Geometry: final body of the model. Coordinates: model frame, mm. Face numbers are marked on the shaded views. Give positions to 0.01 mm unless a question says otherwise; leave off trailing zeros. Loops run counter-clockwise (first coordinate to the right, second up) from the corner with the lowest first, then second, coordinate; pieces in that order, holes last. Notation, with made-up numbers: M -17,64 L 35,64 A16 cw 35,73 Z; hole C 69.25,84.25 d8. An arc over 180 degrees is marked long. Put each result on its own line as item: value.
```python
from build123d import *

# Parameters (mm, degrees)
SKETCH1_R         = 3.175
CENTER_ROD_DEPTH  = 119.888
CIRCLE_ENDS_DEPTH = 3.175


with BuildPart() as part:
    # Sketch1 → center rod (new body)
    with BuildSketch(Plane(origin=(0, 0, 0), x_dir=(1, 0, 0), z_dir=(0, 1, 0))):
        with Locations(Location((0, 0, 0), (0, 0, 270))):
            Circle(SKETCH1_R)
    extrude(amount=CENTER_ROD_DEPTH)

    # Sketch2 → circle ends (add, symmetric)
    with BuildSketch(Plane.XY):
        with BuildLine():
            Line((-3.175, 119.888), (3.175, 119.888))
            ThreePointArc((3.175, 119.888), (0, 131.737261314), (-3.175, 119.888))
        make_face()
        with BuildLine():
            Line((-3.175, 0), (3.175, 0))
            ThreePointArc((3.175, 0), (0, -11.849261314), (-3.175, 0))
        make_face()
    extrude(amount=CIRCLE_ENDS_DEPTH, both=True)


solid = part.part
```
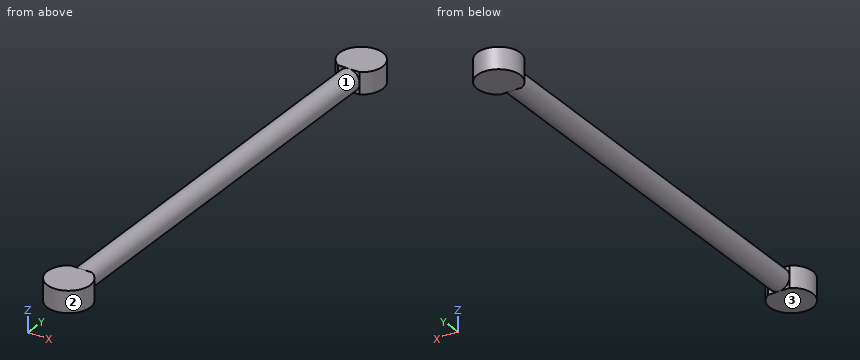
Item 1: Section A-A on x = -5. Output: boundary loops of the cut face in (y, z) (3 decimals), then the cut area to 3 significant figures.
Output values:
outline: M -9.414,-3.175 L -1.585,-3.175 L -1.585,3.175 L -9.414,3.175 Z; M 121.473,-3.175 L 129.302,-3.175 L 129.302,3.175 L 121.473,3.175 Z
area: 99.4 mm²
Item 2: Section B-B on y = 67. Output: boundary loops of the cut face in (x, z) (3 decimals).
Output values:
outline: C 0,0 d6.35
Item 3: Pin query (flat end, axial travel): pin 1 Ø1 at (x, z) = (-1.5, 1) entering from -Y; pin 2 Ø1.6 at (x, z) = (-1.5, -2.5) entering from +Y; pin 3 Ø1 at (x, z) = (2, -2.5) entering from -Y. Return the tip coordinate at first contact, or that it passes through.
Output values:
pin 1: y = -11.77
pin 2: y = 131.7
pin 3: y = -11.67
Item 4: Mould query, pull axis Y, two halves, no side actions, for the marked faces 1, 2 and 3. Classes: pulls with the +Y half, pulls with the -Y half, needs draft (parallel to the pull), parting line crosses it, or undercut.
Output values:
face 1: undercut
face 2: undercut
face 3: needs draft
Item 5: Line query: probe 1 along Y at (x, z) = (5.5, -0.25); probe 2 along Y at (x, z) = (4.5, -0.5); probe 3 along Z at (x, y) = (0.25, 23.5). Output: solid intervals per line, ascending. Write a range as [from, to].
Output values:
probe 1: [-8.67, -2.33], [122.21, 128.56]
probe 2: [-9.98, -1.02], [120.91, 129.87]
probe 3: [-3.17, 3.17]
Item 6: Section C-C on z = -2. Output: boundary loops of the cut face in (x, y) (3 decimals), then the cut area to 3 significant figures.
Output values:
outline: M -3.175,0 A6.35 ccw long 3.175,0 L 2.466,0 L 2.466,119.888 L 3.175,119.888 A6.35 ccw long -3.175,119.888 L -2.466,119.888 L -2.466,0 Z
area: 837 mm²
